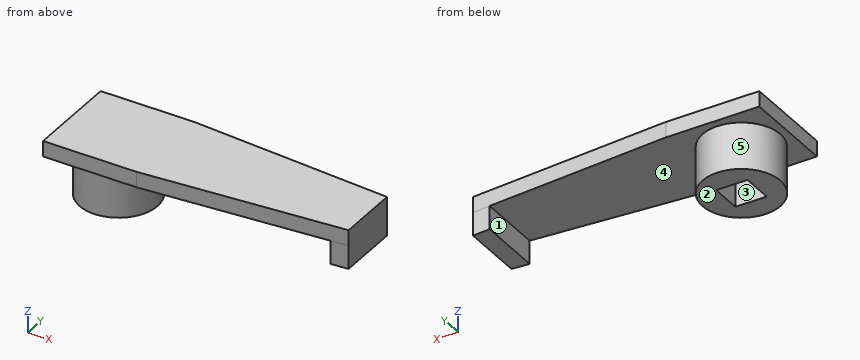
```python
from build123d import *

# Parameters (mm, degrees)
SKETCH2_R           = 12.5
BOSS_EXTRUDE1_DEPTH = 15
SKETCH3_W           = 30
SKETCH3_H           = 30
BOSS_EXTRUDE2_DEPTH = 5
SKETCH6_W           = 10
SKETCH6_H           = 10
CUT_EXTRUDE1_DEPTH  = 15
BOSS_EXTRUDE3_DEPTH = 7.5


with BuildPart() as part:
    # Sketch2 → Boss-Extrude1 (new body)
    with BuildSketch(Plane.XY):
        Circle(SKETCH2_R)
    extrude(amount=BOSS_EXTRUDE1_DEPTH)

    # Sketch3 → Boss-Extrude2 (add)
    with BuildSketch(Plane.XY.offset(15)):
        Rectangle(SKETCH3_W, SKETCH3_H)
    extrude(amount=BOSS_EXTRUDE2_DEPTH)

    # Sketch5 → Loft1 section 0
    with BuildSketch(Plane(origin=(15, 0, 0), x_dir=(0, 0, -1), z_dir=(1, 0, 0))):
        with BuildLine():
            Line((-20, 15), (-15, 15))
            Line((-15, 15), (-15, -15))
            Line((-15, -15), (-20, -15))
            Line((-20, -15), (-20, 15))
        make_face()
    # Sketch4 → Loft1 section 1
    with BuildSketch(Plane(origin=(80, 0, 0), x_dir=(0, 0, -1), z_dir=(1, 0, 0))):
        with BuildLine():
            Line((-20, 10), (-15, 10))
            Line((-15, 10), (-15, -10))
            Line((-15, -10), (-20, -10))
            Line((-20, -10), (-20, 10))
        make_face()
    loft()

    # Sketch6 → Cut-Extrude1 (cut)
    with BuildSketch(Plane(origin=(0, 0, 0), x_dir=(-1, 0, 0), z_dir=(0, 0, -1))):
        Rectangle(SKETCH6_W, SKETCH6_H)
    extrude(amount=-CUT_EXTRUDE1_DEPTH, mode=Mode.SUBTRACT)

    # Sketch7 → Boss-Extrude3 (add)
    with BuildSketch(Plane(origin=(0, 0, 15), x_dir=(-1, 0, 0), z_dir=(0, 0, -1))):
        Polygon((-74.407472361, 10.430194434), (-74.407472361, -10.430194434), (-80, -10), (-80, 10), align=None)
    extrude(amount=BOSS_EXTRUDE3_DEPTH)


solid = part.part
```
Here's how the part is built. I have some questions about the finished solid (model axes, mm). Face numbers are marked on the shaded views. A direction names the side the tool comes from. Round coordinates to 2 decimals unless told otherwise and drop trailing zeros. Order: outer loops, then holes, each group sorted by start corner. A loop starts at its lowest first (then second) coordinate and runs counter-clockwise, first axis right, second up. Notation, with made-up numbers: (51.25, 40) -> (72.25, 40) arc R21 cw to (72.25, 78) -> close; hole circle Ø4 at (4, 84.25). An arc over 180 degrees is marked (long way). Use a Markdown table: item, result. Add a question column.
(1) Suppose I cut it at B-B, the plane x = 0. Please give me the cut outline in (y, z), and give its area (3 significant figures).
(2) If we mould it in two halves opening along Y, with no side actions, what happens to the marked faces 3, 4 and 5? For each: released by +Y, released by -Y, zero draft, split by the parting line, or undercut.
(3) For pin 1 Ø5 at (x, z) = (1, 4) entering from +Y; pin 2 Ø8 at (x, z) = (2, 4) entering from -Y; pin 3 Ø4 at (y, z) = (10.5, 3.5) entering from +X, each with a flat end and sliding along its axis, tell me the tip position at first contact or that it passes through.
(4) I need wall thicknesses on line 1 along X through (y, z) = (0.5, 9.25); line 2 along Z through (x, y) = (66.5, 9); line 3 along X through (y, z) = (-8.5, 13.25). Which ranges of each line are inside material? Lowest first, please.
(5) For the marked faces 1 and 2, which set-ups out of +Z, -Z, +X, -X, +Y, -Y let a thin tool reach every point of the face, with its end or its side?
(6) Suppose I cut it at C-C, the plane y = 0. Please give me the cut outline in (x, z), and give its area (3 significant figures).
(7) Suppose I cut it at A-A, the plane z = 12.25. Please give me the cut outline in (x, y).
(8) Suppose I cut it at D-D, the plane z = 17.25. Please give me the cut outline in (x, y), and give its area (4 significant figures).
Verdict:
| question | item | result |
|---|---|---|
| 1 | outline | (-15, 15) -> (-12.5, 15) -> (-12.5, 0) -> (-5, 0) -> (-5, 15) -> (5, 15) -> (5, 0) -> (12.5, 0) -> (12.5, 15) -> (15, 15) -> (15, 20) -> (-15, 20) -> close |
| 1 | area | 375 mm2 |
| 2 | face 3 | undercut |
| 2 | face 4 | zero draft |
| 2 | face 5 | split by the parting line |
| 3 | pin 1 | y = 12.5 |
| 3 | pin 2 | y = -12.5 |
| 3 | pin 3 | x = 9.17 |
| 4 | line 1 | -12.49 to -5, 5 to 12.49, 74.41 to 80 |
| 4 | line 2 | 15 to 20 |
| 4 | line 3 | -9.17 to 9.17, 74.41 to 80 |
| 5 | face 1 | -Z, +Y, -Y |
| 5 | face 2 | -Z, +X, -X, +Y, -Y |
| 6 | outline | (-15, 15) -> (-12.5, 15) -> (-12.5, 0) -> (-5, 0) -> (-5, 15) -> (5, 15) -> (5, 0) -> (12.5, 0) -> (12.5, 15) -> (74.41, 15) -> (74.41, 7.5) -> (80, 7.5) -> (80, 20) -> (-15, 20) -> close |
| 6 | area | 742 mm2 |
| 7 | outline | circle Ø25 at (0, 0); (74.41, -10.43) -> (80, -10) -> (80, 10) -> (74.41, 10.43) -> close; hole (-5, -5) -> (5, -5) -> (5, 5) -> (-5, 5) -> close |
| 8 | outline | (-15, -15) -> (15, -15) -> (80, -10) -> (80, 10) -> (15, 15) -> (-15, 15) -> close |
| 8 | area | 2,525 mm2 |
